Input: dimensioned drawing with shaded views. Units: mm. Origin: part minimum x, y, z. Give positions to 0.01 mm unless a question says otherwise; leave off trailing zeros. Write each loop counter-clockwise with the first axis right and the second up, starting at its lowest first coordinate (ties: lowest second). Pieces come first, ordered by that corner, then holes. Notation, with made-up numbers: M -23.75,31 L 8.25,31 A22 ccw 8.25,67 Z; hole C 86,-37 d5. An arc over 180 degrees is marked long. Answer as a JSON object with one key per item and string values.
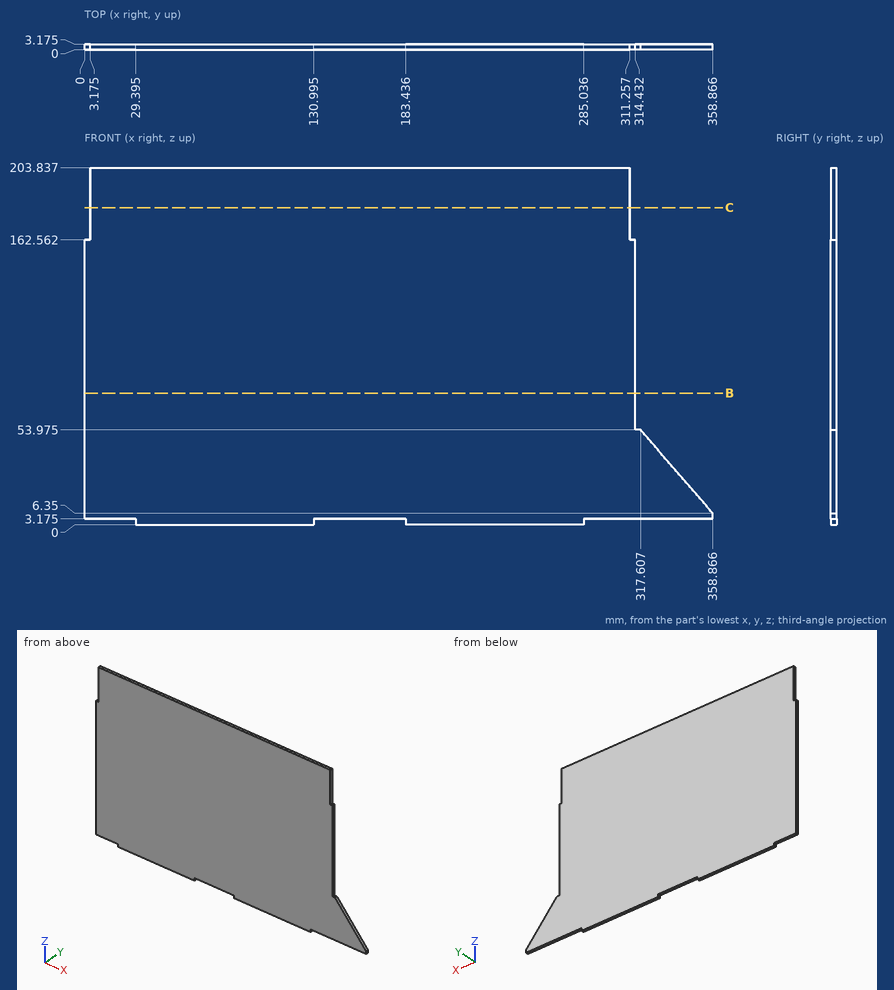
1) Contact query for flat-ended pins moving along their axis: P1, Ø1.6, axis at x = 312.5, y = 1.5, coming from the +Z side; P2, Ø1.6, axis at y = 2, z = 132.5, coming from the +X side; P3, Ø1, axis at x = 164, y = 1, coming from the -Z side (3 decimals). Output: stop coordinate, or through.
Geometry check:
{"P1": "stops at z = 162.56", "P2": "stops at x = 314.43", "P3": "stops at z = 3.175"}
2) Cut plane C-C on z = 181. Return loops of the section in (x, y) (1 decimal).
Geometry check:
{"outline": "M 3.2,0 L 311.3,0 L 311.3,3.2 L 3.2,3.2 Z"}
3) Cut plane B-B on z = 75. Return loops of the section in (x, y) (1 decimal).
Geometry check:
{"outline": "M 0,0 L 314.4,0 L 314.4,3.2 L 0,3.2 Z"}
4) Line query: line 1 (X direction, y = 0.6, z = 107); line 2 (Z direction, x = 149, y = 1.9) (1 decimal); line 3 (X direction, y = 2, z = 195) (1 decimal). Output: solid intervals per line, ascending. Write a range as from..to.
Geometry check:
{"line 1": "x = 0..314.43", "line 2": "z = 3.2..203.8", "line 3": "x = 3.2..311.3"}
